Could you check a few things on this model? Use its own coordinates, in mm. Face numbers are marked on the shaded views. A direction names the side the tool comes from. Coordinates: 2 decimals unless noted, no trailing zeros. Loops run counter-clockwise (first coordinate to the right, second up) from the corner with the lowest first, then second, coordinate; pieces in that order, holes last. Notation, with made-up numbers: (4, 17) - (28, 17) arc R16 cw to (28, 28) - close; hole circle Ø7 at (-24, -21). An arc over 180 degrees is marked (long way). Put each result on its own line as item: value. Start each with the question number.
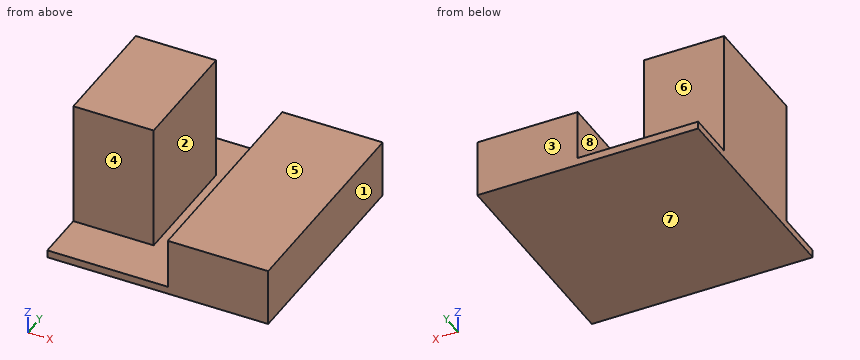
Autodesk Fusion 360 part; units mm, degrees
sketch "Esquisse1" plane through (0, 0, 0) normal (0, 0, 1) x (1, 0, 0)
  line L0 (0, 0) -> (4.4, 0)
  line L1 (4.4, 0) -> (4.4, 4.4)
  line L2 (4.4, 4.4) -> (0, 4.4)
  line L3 (0, 4.4) -> (0, 0)
  dimension "d1" = 4.4
  dimension "d2" = 4.4
extrude "Extrusion1" add sketch "Esquisse1" along normal blind 0.15
sketch "Esquisse2" plane through (0, 0, 0.15) normal (0, 0, 1) x (-1, 0, 0)
  line L0 (0, -4.4) -> (0, 0)
  line L1 (0, 0) -> (-4.4, 0)
  line L2 (-4.4, 0) -> (-4.4, -4.4)
  line L3 (-4.4, -4.4) -> (0, -4.4)
  line L4 (-4.4, 0) -> (-2.4, 0)
  line L5 (-2.4, 0) -> (-2.4, -4.4)
  line L6 (-2.4, -4.4) -> (-4.4, -4.4)
  line L7 (-4.4, -4.4) -> (-4.4, 0)
  dimension "d5" = 2
extrude "Extrusion2" add sketch "Esquisse2" along normal blind 1 contours L1 L2 L3 L4 L5 L6 L7
sketch "Esquisse3" plane through (0, 0, 0.15) normal (0, 0, 1) x (-1, 0, 0)
  line L0 (-2.4, 0) -> (-2.4, -4.4)
  line L1 (-2.4, -4.4) -> (0, -4.4)
  line L2 (0, -4.4) -> (0, 0)
  line L3 (0, 0) -> (-2.4, 0)
  line L4 (0, -3.4) -> (-1.6, -3.4)
  line L5 (-1.6, -3.4) -> (-1.6, -1)
  line L6 (-1.6, -1) -> (0, -1)
  line L7 (0, -1) -> (0, -3.4)
  dimension "d8" = 1.6
  dimension "d9" = 2.4
  dimension "d11" = 1
extrude "Extrusion3" add sketch "Esquisse3" along normal blind 2.5 contours L2 L4 L5 L6 L7
scale "Echelle1" factor 10 about (0, 3.4, 2.65) bodies 1
(1) I want a section at B-B on x = 13. List the corners of the cut face in (y, z) for me.
(2) If we mould it in two halves opening along X, with no side actions, what happens to the marked faces 1, 2 and 3? For each: pulls with the +X half, pulls with the -X half, needs draft (parallel to the pull), parting line crosses it, or undercut.
(3) Which directions (+Z, -Z, +X, -X, +Y, -Y) give clear straight access to the entire face, cutting with the end or side of a thin tool? Please do the marked faces 4, 5, 6, 7 and 8.
(4) I want a section at A-A on z = -21.75. List the corners of the cut face in (x, y) for me.
(5) For pin 1 Ø1 at (x, y) = (21.5, -14.5) entering from +Z; pin 2 Ø5 at (x, z) = (8.5, -6.5) entering from +Y; pin 3 Ø8 at (x, z) = (4, -13.5) entering from -Y, each with a flat end and sliding along its axis, tell me the tip position at first contact or that it passes through.
(6) I want a section at C-C on y = -19. List the corners of the cut face in (x, z) for me, and give its area (3 significant figures).
(7) I want a section at D-D on z = -2.5. List the corners of the cut face in (x, y) for me, and give its area (3 significant figures).
(8) I need wall thicknesses on L1, parallel to X at y = -4, z = -19.75; L2, parallel to X at y = 3.5, z = -17.5; L3, parallel to Z at x = 24.5, y = 9.5. Which ranges of each line are inside material? Lowest first, please. Write a range as [from, to].
Answer sheet:
1. outline: (-30.6, -23.85) - (13.4, -23.85) - (13.4, -22.35) - (3.4, -22.35) - (3.4, 2.65) - (-20.6, 2.65) - (-20.6, -22.35) - (-30.6, -22.35) - close
2. face 1: pulls with the +X half
2. face 2: undercut
2. face 3: needs draft
3. face 4: +Z, -X, -Y
3. face 5: +Z, +X, +Y, -Y
3. face 6: +Z, -X, +Y
3. face 7: -Z, +X, -X, +Y, -Y
3. face 8: +Z, +Y, -Y
4. outline: (0, -20.6) - (16, -20.6) - (16, 3.4) - (0, 3.4) - close; (24, -30.6) - (44, -30.6) - (44, 13.4) - (24, 13.4) - close
5. pin 1: stops at z = -22.35
5. pin 2: stops at y = 3.4
5. pin 3: stops at y = -20.6
6. outline: (0, -23.85) - (44, -23.85) - (44, -12.35) - (24, -12.35) - (24, -22.35) - (16, -22.35) - (16, 2.65) - (0, 2.65) - close
6. area: 666 mm^2
7. outline: (0, -20.6) - (16, -20.6) - (16, 3.4) - (0, 3.4) - close
7. area: 384 mm^2
8. L1: x = [0, 16], [24, 44]
8. L2: x = [24, 44]
8. L3: z = [-23.85, -12.35]
